Geometry check sheet. Reference: the model listing, model coordinates, mm. Round coordinates to 2 decimals unless told otherwise and drop trailing zeros. Order: outer loops, then holes, each group sorted by start corner. A loop starts at its lowest first (then second) coordinate and runs counter-clockwise, first axis right, second up.
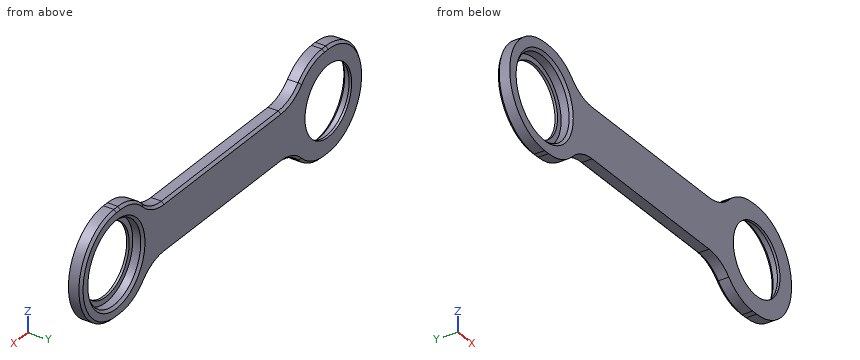
```python
from build123d import *

# Parameters (mm, degrees)
SKETCH1_R           = 16.15
BOSS_EXTRUDE1_DEPTH = 5.2
FILLET1_R           = 20
CHAMFER1_SIZE       = 1
SKETCH2_R           = 19.025242353
SKETCH2_R_2         = 14
BOSS_EXTRUDE2_DEPTH = 1
SKETCH4_R           = 18.71529055
SKETCH4_R_2         = 14
BOSS_EXTRUDE3_DEPTH = 1
CHAMFER2_SIZE       = 1


with BuildPart() as part:
    # Sketch1 → Boss-Extrude1 (new body)
    with BuildSketch(Plane(origin=(0, 0, 0), x_dir=(1, 0, 0), z_dir=(0, 1, 0))):
        with BuildLine():
            Line((50.6952797, -21), (63.625, -21))
            ThreePointArc((63.625, -21), (84.625, 0), (63.625, 21))
            Line((63.625, 21), (50.6952797, 21))
            ThreePointArc((50.6952797, 21), (44.646090821, 13.026866227), (35.106613419, 10))
            Line((35.106613419, 10), (-35.106613419, 10))
            ThreePointArc((-35.106613419, 10), (-44.646090821, 13.026866227), (-50.6952797, 21))
            Line((-50.6952797, 21), (-63.625, 21))
            ThreePointArc((-63.625, 21), (-84.625, 0), (-63.625, -21))
            Line((-63.625, -21), (-50.6952797, -21))
            ThreePointArc((-50.6952797, -21), (-44.646090821, -13.026866227), (-35.106613419, -10))
            Line((-35.106613419, -10), (35.106613419, -10))
            ThreePointArc((35.106613419, -10), (44.646090821, -13.026866227), (50.6952797, -21))
        make_face()
        with Locations((-63.625, 0)):
            Circle(SKETCH1_R, mode=Mode.SUBTRACT)
        with Locations((63.625, 0)):
            Circle(SKETCH1_R, mode=Mode.SUBTRACT)
    extrude(amount=BOSS_EXTRUDE1_DEPTH)

    # Fillet1
    fillet1_edges = [part.edges().sort_by_distance(p)[0] for p in [
        (-50.6952797, 2.6, 21),
        (-50.6952797, 2.6, -21),
        (50.6952797, 2.6, -21),
        (50.6952797, 2.6, 21),
    ]]
    fillet(fillet1_edges, radius=FILLET1_R)

    # Chamfer1
    chamfer1_edges = [part.edges().sort_by_distance(p)[0] for p in [
        (62.433003391, 5.2, 21),
        (84.625, 5.2, 0),
        (62.433003391, 5.2, -21),
        (41.52534742, 5.2, -11.295776268),
        (0, 5.2, -10),
        (41.52534742, 5.2, 11.295776268),
        (-41.52534742, 5.2, -11.295776268),
        (-62.433003391, 5.2, -21),
        (-62.433003391, 5.2, 21),
        (-53.482236449, 5.2, 19.433705079),
        (-53.482236449, 5.2, -19.433705079),
        (-84.625, 5.2, 0),
        (53.482236449, 5.2, -19.433705079),
        (53.482236449, 5.2, 19.433705079),
        (-41.52534742, 5.2, 11.295776268),
        (0, 5.2, 10),
        (47.475, 5.2, 0),
    ]]
    chamfer(chamfer1_edges, length=CHAMFER1_SIZE)

    # Sketch2 → Boss-Extrude2 (add)
    with BuildSketch(Plane.XZ):
        with Locations((63.625, 0)):
            Circle(SKETCH2_R)
        with Locations((63.625, 0)):
            Circle(SKETCH2_R_2, mode=Mode.SUBTRACT)
    extrude(amount=-BOSS_EXTRUDE2_DEPTH)

    # Sketch4 → Boss-Extrude3 (add)
    with BuildSketch(Plane(origin=(0, 5.2, 0), x_dir=(1, 0, 0), z_dir=(0, 1, 0))):
        with Locations((-63.625, 0)):
            Circle(SKETCH4_R)
        with Locations((-63.625, 0)):
            Circle(SKETCH4_R_2, mode=Mode.SUBTRACT)
    extrude(amount=-BOSS_EXTRUDE3_DEPTH)

    # Chamfer2
    chamfer2_edges = [part.edges().sort_by_distance(p)[0] for p in [
        (-79.775, 0, 0),
    ]]
    chamfer(chamfer2_edges, length=CHAMFER2_SIZE)


solid = part.part
```
(1) Depth check by flat-ended pin: P1, Ø3, axis at x = 66, y = 3, coming from the +Z side; P2, Ø2, axis at x = 8.5, y = 1.5, coming from the -Z side; P3, Ø25, axis at x = -63.625, z = 0, coming from the +Y side (3 decimals); P4, Ø16, axis at x = -70, z = -3.5, coming from the -Y side. Enter the tip coordinate at first touch or a pass-through.
Returned:
P1: stops at z = 20.98
P2: stops at z = -10
P3: passes through
P4: stops at y = 4.2
(2) Sectioned sample at C-C, the plane x = -29. Record the cut outline in (y, z), and give its area (3 significant figures).
Returned:
outline: (0, -10) - (4.2, -10) - (5.2, -9) - (5.2, 9) - (4.2, 10) - (0, 10) - close
area: 103 mm2
(3) Sectioned sample at B-B, the plane y = 1.8. Give the number of separate pieces and of enclosed holes in the cut face, and give its area (3 significant figures).
Returned:
separate pieces: 1
enclosed holes: 2
area: 2,990 mm2
(4) Sectioned sample at A-A, the plane z = 0. Record the cut outline in (x, y) (3 decimals), and give its area (3 significant figures).
Returned:
outline: (-84.625, 0) - (-80.775, 0) - (-79.775, 1) - (-79.775, 4.2) - (-77.625, 4.2) - (-77.625, 5.2) - (-83.625, 5.2) - (-84.625, 4.2) - close; (-49.625, 4.2) - (-47.475, 4.2) - (-47.475, 1) - (-46.475, 0) - (49.625, 0) - (49.625, 1) - (47.475, 1) - (47.475, 4.2) - (46.475, 5.2) - (-49.625, 5.2) - close; (77.625, 0) - (84.625, 0) - (84.625, 4.2) - (83.625, 5.2) - (80.775, 5.2) - (79.775, 4.2) - (79.775, 1) - (77.625, 1) - close
area: 550 mm2
(5) Material ranges on line 1 (X direction, y = 2.15, z = 0) (3 decimals); line 2 (X direction, y = 4.8, z = 0) (3 decimals); line 3 (Z direction, x = -25, y = 0.75), recorded low to high.
Returned:
line 1: x = -84.625 to -79.775, -47.475 to 47.475, 79.775 to 84.625
line 2: x = -84.025 to -77.625, -49.625 to 46.875, 80.375 to 84.025
line 3: z = -10 to 10
